```python
from build123d import *

# Parameters (mm, degrees)
SKETCH_1_W                = 80
SKETCH_1_H                = 80
EXTRUDE_1_DEPTH           = 11
FILLET_1_R                = 20
FILLET_2_R                = 5
SKETCH_2_W                = 30
SKETCH_2_H                = 15
CUT_EXTRUDE_1_DEPTH       = 11
FILLET_3_R                = 2
SKETCH_3_W                = 35.5
SKETCH_3_H                = 6
CUT_EXTRUDE_2_DEPTH       = 11
SKETCH_4_W                = 35.5
SKETCH_4_H                = 6
CUT_EXTRUDE_3_DEPTH       = 11
SKETCH_5_W                = 5
SKETCH_5_H                = 40
CUT_EXTRUDE_4_DEPTH       = 11
FILLET_4_R                = 2
SKETCH_8_R                = 1.9
CUT_EXTRUDE_5_DEPTH       = 11
CUT_EXTRUDE_6_DEPTH       = 8.5
EXTRUDE_2_DEPTH           = 6.2
HOLE_WIZARD_2_D           = 6.6
HOLE_WIZARD_2_CBORE_D     = 11
HOLE_WIZARD_2_CBORE_DEPTH = 6.8


with BuildPart() as part:
    # 草图1 → 凸台-拉伸1 (new body)
    with BuildSketch(Plane.XY):
        with Locations((3.759980536, -13.590563907)):
            Rectangle(SKETCH_1_W, SKETCH_1_H)
    extrude(amount=EXTRUDE_1_DEPTH)

    # 圆角1
    fillet_1_edges = [part.edges().sort_by_distance(p)[0] for p in [
        (-36.240019464, 26.409436093, 5.5),
        (-36.240019464, -53.590563907, 5.5),
    ]]
    fillet(fillet_1_edges, radius=FILLET_1_R)

    # 圆角2
    fillet_2_edges = [part.edges().sort_by_distance(p)[0] for p in [
        (43.759980536, 26.409436093, 5.5),
        (43.759980536, -53.590563907, 5.5),
    ]]
    fillet(fillet_2_edges, radius=FILLET_2_R)

    # 草图2 → 切除-拉伸1 (cut)
    with BuildSketch(Plane(origin=(0, 0, 0), x_dir=(-1, 0, 0), z_dir=(0, 0, -1))):
        with Locations((21.240019464, -13.590563907)):
            Rectangle(SKETCH_2_W, SKETCH_2_H)
    extrude(amount=-CUT_EXTRUDE_1_DEPTH, mode=Mode.SUBTRACT)

    # 圆角3
    fillet_3_edges = [part.edges().sort_by_distance(p)[0] for p in [
        (-36.240019464, -6.090563907, 5.5),
        (-36.240019464, -21.090563907, 5.5),
        (-6.240019464, -21.090563907, 5.5),
        (-6.240019464, -6.090563907, 5.5),
    ]]
    fillet(fillet_3_edges, radius=FILLET_3_R)

    # 草图3 → 切除-拉伸2 (cut)
    with BuildSketch(Plane.XY.offset(11)):
        with Locations((14.009980536, 23.409436093)):
            Rectangle(SKETCH_3_W, SKETCH_3_H)
    extrude(amount=-CUT_EXTRUDE_2_DEPTH, mode=Mode.SUBTRACT)

    # 草图4 → 切除-拉伸3 (cut)
    with BuildSketch(Plane.XY.offset(11)):
        with Locations((14.009980536, -50.590563907)):
            Rectangle(SKETCH_4_W, SKETCH_4_H)
    extrude(amount=-CUT_EXTRUDE_3_DEPTH, mode=Mode.SUBTRACT)

    # 草图5 → 切除-拉伸4 (cut)
    with BuildSketch(Plane.XY.offset(11)):
        with Locations((41.259980536, -13.590563907)):
            Rectangle(SKETCH_5_W, SKETCH_5_H)
    extrude(amount=-CUT_EXTRUDE_4_DEPTH, mode=Mode.SUBTRACT)

    # 圆角4
    fillet_4_edges = [part.edges().sort_by_distance(p)[0] for p in [
        (43.759980536, 6.409436093, 5.5),
        (41.259980536, -33.590563907, 0),
        (43.759980536, -33.590563907, 5.5),
        (38.759980536, -13.590563907, 0),
        (38.759980536, -33.590563907, 5.5),
        (41.259980536, 6.409436093, 0),
        (38.759980536, 6.409436093, 5.5),
        (41.259980536, 6.409436093, 11),
        (38.759980536, -13.590563907, 11),
        (41.259980536, -33.590563907, 11),
    ]]
    fillet(fillet_4_edges, radius=FILLET_4_R)

    # 草图8 → 切除-拉伸5 (cut)
    with BuildSketch(Plane.XY.offset(11)):
        with Locations((39.009980536, -41.590563907)):
            Circle(SKETCH_8_R)
        with Locations((-10.990019464, -27.090563907)):
            Circle(SKETCH_8_R)
        with Locations((-10.990019464, -0.090563907)):
            Circle(SKETCH_8_R)
        with Locations((39.009980536, 14.409436093)):
            Circle(SKETCH_8_R)
    extrude(amount=-CUT_EXTRUDE_5_DEPTH, mode=Mode.SUBTRACT)

    # 草图9 → 切除-拉伸6 (cut)
    with BuildSketch(Plane.XY.offset(11)):
        Polygon((-14.890383234, -26.550845651), (-13.40761107, -30.198518888), (-9.5072473, -30.738237144), (-7.089655694, -27.630282164), (-8.572427858, -23.982608927), (-12.472791628, -23.442890671), align=None)
        Polygon((37.527208372, -37.942890671), (35.109616766, -41.050845651), (36.59238893, -44.698518888), (40.4927527, -45.238237144), (42.910344306, -42.130282164), (41.427572142, -38.482608927), align=None)
        Polygon((-8.572427858, 3.017391073), (-12.472791628, 3.557109329), (-14.890383234, 0.449154349), (-13.40761107, -3.198518888), (-9.5072473, -3.738237144), (-7.089655694, -0.630282164), align=None)
        Polygon((36.59238893, 11.301481112), (40.4927527, 10.761762856), (42.910344306, 13.869717836), (41.427572142, 17.517391073), (37.527208372, 18.057109329), (35.109616766, 14.949154349), align=None)
    extrude(amount=-CUT_EXTRUDE_6_DEPTH, mode=Mode.SUBTRACT)

    # 草图10 → 凸台-拉伸2 (add)
    with BuildSketch(Plane.XY.offset(11)):
        with BuildLine():
            Line((-0.740019464, -13.590563907), (-6.895850028, 0.960922273))
            ThreePointArc((-6.895850028, 0.960922273), (15.059980536, -13.590563907), (-6.895850028, -28.142050088))
            Line((-6.895850028, -28.142050088), (-0.740019464, -13.590563907))
        make_face()
    extrude(amount=EXTRUDE_2_DEPTH)

    # 打孔尺寸(%根据)内六角圆柱头螺钉的类型2 (through all)
    with Locations(Plane(origin=(0, 0, 0), x_dir=(-1, 0, 0), z_dir=(0, 0, -1))):
        with Locations((-17.291203456, 4.440659013), (18.771242384, 4.440659013), (18.771242384, -31.621786828), (-17.291203456, -31.621786828)):
            CounterBoreHole(HOLE_WIZARD_2_D / 2, HOLE_WIZARD_2_CBORE_D / 2, HOLE_WIZARD_2_CBORE_DEPTH)


solid = part.part
```
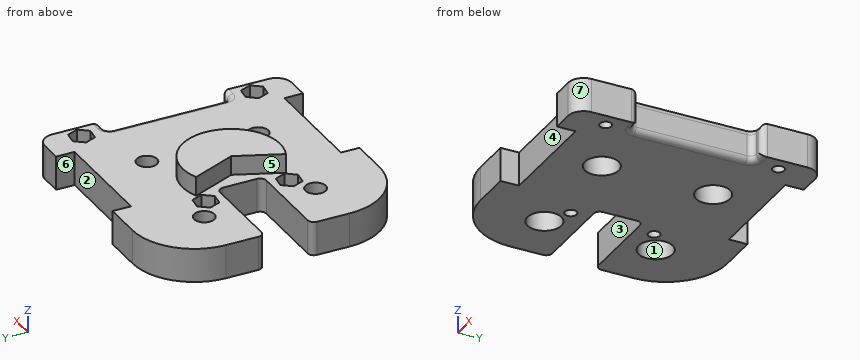
Design review of the part built by this model. Coordinates are the model's own, in mm. Face numbers are marked on the shaded views. A direction names the side the tool comes from. Round coordinates to 2 decimals unless told otherwise and drop trailing zeros. Write each loop counter-clockwise with the first axis right and the second up, starting at its lowest first coordinate (ties: lowest second). Pieces come first, ordered by that corner, then holes. Notation, with made-up numbers: (74, 14) -> (92, 14) arc R16 ccw to (92, 41) -> close; hole circle Ø2 at (66.25, -38). An arc over 180 degrees is marked (long way). Answer in a Markdown table with one row per item.
Q1. Take a section at D-D, the plane y = -10. State the section outline as (x, z) points, then the cut area to 3 significant figures.
The answers:
| item | result |
|---|---|
| outline | (-6.24, 0) -> (36.76, 0) arc R2 ccw to (38.76, 2) -> (38.76, 9) arc R2 ccw to (36.76, 11) -> (14.65, 11) -> (14.65, 17.2) -> (-2.26, 17.2) -> (-2.26, 11) -> (-6.24, 11) -> close |
| area | 598 mm² |
Q2. Take a section at B-B, the plane z = 14. State the section outline as (x, y) points.
The answers:
| item | result |
|---|---|
| outline | (-6.9, -28.14) arc R15.8 ccw (long way) to (-6.9, 0.96) -> (-0.74, -13.59) -> close |
Q3. To check wall thickness, follow L1, parallel to X at y = 9.5, z = 1.25; L2, parallel to Y at x = 39.5, z = 5; L3, parallel to X at y = -8.5, z = 2.25. State the ranges of each line that lie inside material, in increasing order. Write a range as [from, to].
The answers:
| item | result |
|---|---|
| L1 | [-36, -20.93], [-16.61, 15.13], [19.45, 43.76] |
| L2 | [-53.54, -45.1], [-38.22, -33.14], [5.96, 10.9], [17.78, 26.35] |
| L3 | [-6.24, 38.76] |
Q4. Take a section at C-C, the plane x = 8. State the section outline as (y, z) points.
The answers:
| item | result |
|---|---|
| outline | (-47.59, 0) -> (20.41, 0) -> (20.41, 11) -> (-0.43, 11) -> (-0.43, 17.2) -> (-26.75, 17.2) -> (-26.75, 11) -> (-47.59, 11) -> close |
Q5. Draft analysis for pull direction Y (two halves, no side actions). For the marked faces 5, 6 and 7, state which applies: +Y half, -Y half, draft (parallel to the pull), parting line (faces both ways), or undercut.
The answers:
| item | result |
|---|---|
| face 5 | undercut |
| face 6 | draft |
| face 7 | -Y half |
Q6. Take a section at A-A, the plane x = -11. State the section outline as (y, z) points, then the cut area to 3 significant figures.
The answers:
| item | result |
|---|---|
| outline | (-53.59, 0) -> (-28.99, 0) -> (-28.99, 2.5) -> (-30.53, 2.5) -> (-30.53, 11) -> (-53.59, 11) -> close; (-25.19, 0) -> (-21.09, 0) -> (-21.09, 11) -> (-23.65, 11) -> (-23.65, 2.5) -> (-25.19, 2.5) -> close; (-6.09, 0) -> (-1.99, 0) -> (-1.99, 2.5) -> (-3.53, 2.5) -> (-3.53, 11) -> (-6.09, 11) -> close; (1.81, 0) -> (26.41, 0) -> (26.41, 11) -> (3.35, 11) -> (3.35, 2.5) -> (1.81, 2.5) -> close |
| area | 579 mm² |
Q7. Clearance check with flat-ended pins moving along their axes: pin 1 Ø2 at (x, y) = (38, 15.5) entering from +Z; pin 2 Ø7.5 at (x, y) = (-18.77, -31.62) entering from -Z; pin 3 Ø4 at (y, z) = (-18, 3) entering from -X. State where each tip first meets the part, or that it passes through.
The answers:
| item | result |
|---|---|
| pin 1 | z = 2.5 |
| pin 2 | z = 6.8 |
| pin 3 | x = -6.46 |
Q8. For the marked faces 1, 2, 3 and 4, list the 3-axis set-ups (+Z, -Z, +X, -X, +Y, -Y) from which the entire face can be reached by the end or side of a thin tool; tool diameter is ignored.
The answers:
| item | result |
|---|---|
| face 1 | -Z |
| face 2 | +Z, -Z, +Y |
| face 3 | +Z, -Z, -X |
| face 4 | +Z, -Z, -Y |
